Autodesk Inventor part; units mm, degrees
ref_plane "YZ Plane" through (0, 0, 0) normal (1, 0, 0) x (0, 1, 0)
ref_plane "XZ Plane" through (0, 0, 0) normal (0, 1, 0) x (-1, 0, 0)
ref_plane "XY Plane" through (0, 0, 0) normal (0, 0, 1) x (1, 0, 0)
sketch "Sketch1" plane through (0, 0, 0) normal (0, 1, 0) x (-1, 0, 0)
  line L0 (12.4664, 17.9083) -> (-8.3336, 17.9083)
  line L1 (-8.3336, 17.9083) -> (-8.3336, 0.9083)
  line L2 (-8.3336, 0.9083) -> (12.4664, 0.9083)
  line L3 (12.4664, 0.9083) -> (12.4664, 17.9083)
  line L4 (-8.3336, 15.4583) -> (-7.8336, 15.4583)
  line L5 (-7.8336, 15.4583) -> (-7.8336, 3.3583)
  line L6 (-7.8336, 3.3583) -> (-8.3336, 3.3583)
  line L7 (-8.3336, 3.3583) -> (-8.3336, 15.4583)
  line L8 (6.8664, 17.9083) -> (-5.2336, 17.9083)
  line L9 (-5.2336, 17.9083) -> (-5.2336, 17.4083)
  line L10 (-5.2336, 17.4083) -> (6.8664, 17.4083)
  line L11 (6.8664, 17.4083) -> (6.8664, 17.9083)
  line L12 (6.8664, 0.9083) -> (-5.2336, 0.9083)
  line L13 (-5.2336, 0.9083) -> (-5.2336, 1.4083)
  line L14 (-5.2336, 1.4083) -> (6.8664, 1.4083)
  line L15 (6.8664, 1.4083) -> (6.8664, 0.9083)
  point P0 (0, 0)
  dimension "d0" = 20.8
  dimension "d1" = 17
  dimension "d2" = 0.5
  dimension "d3" = 2.45
  dimension "d4" = 2.45
  dimension "d5" = 3.1
  dimension "d6" = 5.6
  dimension "d7" = 0.5
  dimension "d8" = 0.5
extrude "Extrusion1" add sketch "Sketch1" along normal blind 2 contours L3 L2 L15 L14 L13 L1 L6 L5 L4 L0 L9 L10 L11
extrude "Extrusion2" add sketch "Sketch1" along normal blind 2.5 contours L11 L10 L9 L0
extrude "Extrusion3" add sketch "Sketch1" along normal blind 2.5 contours L4 L5 L6 L1
extrude "Extrusion4" add sketch "Sketch1" along normal blind 2.5 contours L2 L13 L14 L15
equation "\"d4\" = d3"
properties part number "čip"
Geometry: final body of the model. Coordinates: model frame, mm. Round coordinates to 2 decimals unless told otherwise and drop trailing zeros. Write each loop counter-clockwise with the first axis right and the second up, starting at its lowest first coordinate (ties: lowest second). Pieces come first, ordered by that corner, then holes.
Item 1: Pin query (flat end, axial travel): P1, Ø5, axis at x = -8, z = 4, coming from the +Y side; P2, Ø0.6, axis at y = 2.5, z = 18, coming from the -X side. Return the tip coordinate at first contact, or that it passes through.
Item 2: Section query B-B (z = 4.25). Return loops of the section in (x, y), plus the area to 4 significant figures.
Item 3: Section query C-C (x = -7.75). Return loops of the section in (y, z), plus the area to 3 significant figures.
Item 4: Material intervals for L1, parallel to Z at x = 0, y = 2.2; L2, parallel to Y at x = -9.5, z = 15; L3, parallel to X at y = 2.1, z = 12, sorted ascending.
Item 5: Section query A-A (x = 4.75). Return loops of the section in (y, z), plus the area to 3 significant figures.
Completed:
1. P1: stops at y = 2
1. P2: stops at x = -6.87
2. outline: (-12.47, 0) - (8.33, 0) - (8.33, 2.5) - (7.83, 2.5) - (7.83, 2) - (-12.47, 2) - close
2. area: 41.85 mm2
3. outline: (0, 0.91) - (2, 0.91) - (2, 17.91) - (0, 17.91) - close
3. area: 34.0 mm2
4. L1: z = 0.91 to 1.41, 17.41 to 17.91
4. L2: y = 0 to 2
4. L3: x = 7.83 to 8.33
5. outline: (0, 0.91) - (2.5, 0.91) - (2.5, 1.41) - (2, 1.41) - (2, 17.41) - (2.5, 17.41) - (2.5, 17.91) - (0, 17.91) - close
5. area: 34.5 mm2
